Check sheet for the modelled part. Datum: model origin and axes. Units: mm. Coordinates: 2 decimals unless noted, no trailing zeros. Loops run counter-clockwise (first coordinate to the right, second up) from the corner with the lowest first, then second, coordinate; pieces in that order, holes last. Notation, with made-up numbers: (45, -30.75) -> (64, -30.75) arc R7 cw to (64, -23.75) -> close; hole circle Ø6 at (35, -36). An arc over 180 degrees is marked (long way). Use CSV: the item, a comma, the result in double quotes. Start each with the question number.
1. Sectioned sample at C-C, the plane z = 25. Record the cut outline in (x, y).
2. Sectioned sample at A-A, the plane y = 0.75. Record the cut outline in (x, z).
3. Sectioned sample at B-B, the plane x = -53. Record the cut outline in (y, z), and give its area (3 significant figures).
4. Thickness scan on L1, parallel to Z at x = -60.5, y = 1.5; L2, parallel to X at y = 3.5, z = -12.5; L3, parallel to X at y = 3.25, z = 34.5. Record the ranges inside material, lowest first.
Autodesk Inventor part; units mm, degrees
ref_plane "YZ Plane" through (0, 0, 0) normal (1, 0, 0) x (0, 1, 0)
ref_plane "XZ Plane" through (0, 0, 0) normal (0, 1, 0) x (-1, 0, 0)
ref_plane "XY Plane" through (0, 0, 0) normal (0, 0, 1) x (1, 0, 0)
sketch "Sketch1" plane through (0, 0, 0) normal (0, 1, 0) x (-1, 0, 0)
  line L0 (45, 42.5) -> (-45, 42.5)
  line L1 (-45, 42.5) -> (-45, -42.5)
  line L2 (-45, -42.5) -> (45, -42.5)
  line L3 (45, 42.5) -> (-45, -42.5) construction
  line L4 (-45, 42.5) -> (45, -42.5) construction
  line L5 (45, 42.5) -> (85, 0)
  line L6 (85, 0) -> (45, -42.5)
  point P0 (0, 0)
  dimension "d0" = 90
  dimension "d1" = 85
extrude "Extrusion1" add sketch "Sketch1" along normal blind 5
properties part number "lidar_base"
Completed:
1,outline,"(-61.47, 0) -> (45, 0) -> (45, 5) -> (-61.47, 5) -> close"
2,outline,"(-85, 0) -> (-45, -42.5) -> (45, -42.5) -> (45, 42.5) -> (-45, 42.5) -> close"
3,outline,"(0, -34) -> (5, -34) -> (5, 34) -> (0, 34) -> close"
3,area,"340 mm²"
4,L1,"-26.03 to 26.03"
4,L2,"-73.24 to 45"
4,L3,"-52.53 to 45"
